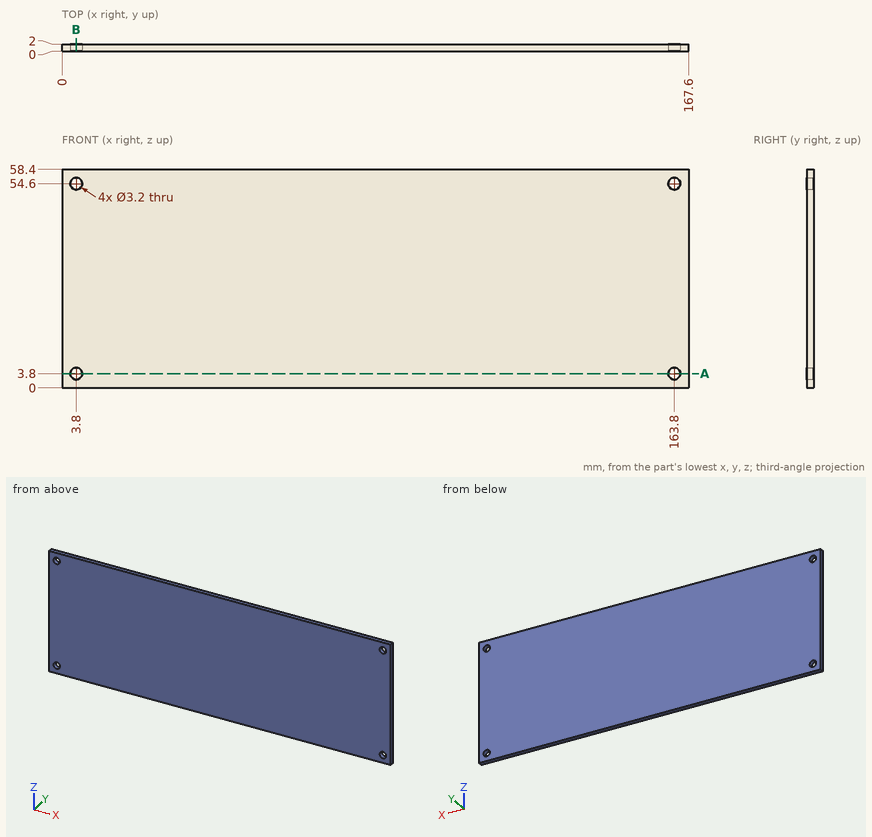
Answer from the drawing. Dimensions are ordinates in mm from the lowest x, y and z of the part. Coordinates: 2 decimals unless noted, no trailing zeros. Write each loop counter-clockwise with the first axis right and the second up, starting at its lowest first coordinate (ties: lowest second). Pieces come first, ordered by that corner, then holes. Notation, with made-up numbers: (30.5, 48.5) - (52.5, 48.5) arc R23 cw to (52.5, 69.5) - close; hole circle Ø7 at (81.25, -40). An arc over 180 degrees is marked (long way). Return JSON: item names as keys, results as strings.
1. The part is cut by section A-A on z = 3.8. Determine the outline of the cut face in (x, y), then the cut area to 3 significant figures.
Final values:
{"outline": "(0, 0) - (2.2, 0) - (2.2, 2) - (0, 2) - close; (5.4, 0) - (162.2, 0) - (162.2, 2) - (5.4, 2) - close; (165.4, 0) - (167.6, 0) - (167.6, 2) - (165.4, 2) - close", "area": "322 mm^2"}
2. This flat-tipped pin is pushed along its axis until it touches: pin 1 Ø12 at (x, z) = (147.5, 23.5) entering from -Y. Where does it stop, or does it pass through?
Final values:
{"pin 1": "y = 0"}
3. Consider line 1 along X through (y, z) = (0.65, 3.8); line 2 along Z through (x, y) = (163.8, 1.3). Determine where each line is inside the solid, lowest interval first.
Final values:
{"line 1": "0 to 2.2, 5.4 to 162.2, 165.4 to 167.6", "line 2": "0 to 2.2, 5.4 to 53, 56.2 to 58.4"}
4. The part is cut by section B-B on x = 3.8. Determine the outline of the cut face in (y, z), then the cut area to 3 significant figures.
Final values:
{"outline": "(0, 0) - (2, 0) - (2, 2.2) - (0, 2.2) - close; (0, 5.4) - (2, 5.4) - (2, 53) - (0, 53) - close; (0, 56.2) - (2, 56.2) - (2, 58.4) - (0, 58.4) - close", "area": "104 mm^2"}
